```python
from build123d import *

# Parameters (mm, degrees)
BOSS_EXTRU_1_DEPTH      = 5
ESQUISSE3_W             = 5
ESQUISSE3_H             = 5
BOSS_EXTRU_3_DEPTH      = 10
ESQUISSE2_W             = 5
ESQUISSE2_H             = 10
BOSS_EXTRU_5_DEPTH      = 10.5
ESQUISSE4_W             = 5
ESQUISSE4_H             = 5
ENL_V_MAT_EXTRU_1_DEPTH = 10


with BuildPart() as part:
    # Esquisse1 → Boss.-Extru.1 (new body)
    with BuildSketch(Plane.XY):
        Polygon((0, 0), (0, 26.2), (21.226398658, 0), align=None)
    extrude(amount=BOSS_EXTRU_1_DEPTH)

    # Esquisse3 → Boss.-Extru.3 (add)
    with BuildSketch(Plane.XZ):
        with Locations((18.726398658, 2.5)):
            Rectangle(ESQUISSE3_W, ESQUISSE3_H)
    extrude(amount=BOSS_EXTRU_3_DEPTH)

    # Esquisse2 → Boss.-Extru.5 (add)
    with BuildSketch(Plane.ZY):
        with Locations((2.5, 17)):
            Rectangle(ESQUISSE2_W, ESQUISSE2_H)
    extrude(amount=BOSS_EXTRU_5_DEPTH)

    # Esquisse4 → Enlèv. mat.-Extru.1 (cut)
    with BuildSketch(Plane(origin=(0, 0, 0), x_dir=(-1, 0, 0), z_dir=(0, 0, -1))):
        with Locations((5.5, 17)):
            Rectangle(ESQUISSE4_W, ESQUISSE4_H)
    extrude(amount=-ENL_V_MAT_EXTRU_1_DEPTH, mode=Mode.SUBTRACT)


solid = part.part
```
Part model, mm, in its own coordinate system. A direction names the side the tool comes from. Give positions to 0.01 mm unless a question says otherwise; leave off trailing zeros. Loops run counter-clockwise (first coordinate to the right, second up) from the corner with the lowest first, then second, coordinate; pieces in that order, holes last. Notation, with made-up numbers: M 9,21 L 35,21 A37 cw 35,60 Z; hole C -37,42.25 d11. An arc over 180 degrees is marked long. Return JSON: item names as keys, results as strings.
1) Saw through at A-A, the plane z = 0.95. List the corners of the cut face in (x, y), then the cut area to 3 significant figures.
Calculated:
{"outline": "M -10.5,12 L 0,12 L 0,0 L 16.23,0 L 16.23,-10 L 21.23,-10 L 21.23,0 L 0,26.2 L 0,22 L -10.5,22 Z; hole M -8,14.5 L -3,14.5 L -3,19.5 L -8,19.5 Z", "area": "408 mm2"}
2) Drill centre lines: line 1 (Y direction, x = -3.5, z = 2.15); line 2 (X direction, y = 16, z = 3.8); line 3 (Y direction, x = -9, z = 4.25). Where is each one in solid material? Low to high.
Calculated:
{"line 1": "y = 12 to 14.5, 19.5 to 22", "line 2": "x = -10.5 to -8, -3 to 8.26", "line 3": "y = 12 to 22"}
3) Pull direction X, two halves, no side cores. Call faces 5 (the face through (10.465, 13.283, 2.465)), 6 (the face through (-5, 22, 2)), 7 (the face through (-5, 19.5, 2)): released by +X, released by -X, zero draft, split by the parting line, or undercut.
Calculated:
{"face 5": "released by +X", "face 6": "zero draft", "face 7": "undercut"}
4) Saw through at B-B, the plane y = 16. List the corners of the cut face in (x, z).
Calculated:
{"outline": "M -10.5,0 L -8,0 L -8,5 L -10.5,5 Z; M -3,0 L 8.26,0 L 8.26,5 L -3,5 Z"}
5) 3-axis set-ups, long thin cutter, end or side, ignore diameter. For faces 1 (the face through (0, 24, 2)), 2 (the face through (-3, 17, 2)), 3 (the face through (16.226, -5, 2)), 4 (the face through (-10.5, 17, 2)): which of +Z, -Z, +X, -X, +Y, -Y reach the whole face in a straight line?
Calculated:
{"face 1": "+Z, -Z, -X, +Y", "face 2": "+Z, -Z", "face 3": "+Z, -Z, -X, -Y", "face 4": "+Z, -Z, -X, +Y, -Y"}
6) Saw through at C-C, the plane x = -2. List the corners of the cut face in (y, z).
Calculated:
{"outline": "M 12,0 L 22,0 L 22,5 L 12,5 Z"}
7) Flat gauge pins, fed straight in: pin 1 Ø2.5 at (x, z) = (-7.5, 3.5) entering from -Y; pin 2 Ø2 at (x, z) = (3.5, 2) entering from -Y; pin 3 Ø2.5 at (y, z) = (-5.5, 2.5) entering from -X. Where does each tip first touch, or does it go through?
Calculated:
{"pin 1": "stops at y = 12", "pin 2": "stops at y = 0", "pin 3": "stops at x = 16.23"}
8) Saw through at D-D, the plane y = -7.5. List the corners of the cut face in (x, z), then the cut area to 3 significant figures.
Calculated:
{"outline": "M 16.23,0 L 21.23,0 L 21.23,5 L 16.23,5 Z", "area": "25.0 mm2"}
